Input: part model. Units: mm. Frame: model coordinates. Round coordinates to 2 decimals unless told otherwise and drop trailing zeros. Loops run counter-clockwise (first coordinate to the right, second up) from the corner with the lowest first, then second, coordinate; pieces in that order, holes last. Notation, with made-up numbers: (75, -16) -> (102, -16) arc R25 ccw to (102, 7) -> close; hole circle Ø6 at (86.25, 32). An arc over 180 degrees is marked (long way). Answer as a JSON object with one key per item and string values.
```python
from build123d import *

# Parameters (mm, degrees)
F0_W     = 15
F0_H     = 100
F2_R     = 3.9
F3_DEPTH = 10
F4_R     = 5


with BuildPart() as f1:
    # F0 (on Top) → F1 (revolve)
    with BuildSketch(Plane.XY):
        with Locations((-7.5, -50)):
            Rectangle(F0_W, F0_H)
    revolve(axis=Axis((0, -50, 0), (0, 1, 0)))

    # F2 (on face) → F3 (cut)
    with BuildSketch(Plane(origin=(0, 0, 0), x_dir=(-1, 0, 0), z_dir=(0, 1, 0))):
        Circle(F2_R)
    extrude(amount=-F3_DEPTH, mode=Mode.SUBTRACT)

    # F4
    f4_edges = [f1.edges().sort_by_distance(p)[0] for p in [
        (15, 0, 0),
        (15, -100, 0),
    ]]
    fillet(f4_edges, radius=F4_R)


solid = f1.part
```
1) Section A-A, the plane z = 0. Output: boundary loops of the cut face in (x, y), plus the area to 3 significant figures.
Output:
{"outline": "(-15, -95) arc R5 ccw to (-10, -100) -> (10, -100) arc R5 ccw to (15, -95) -> (15, -5) arc R5 ccw to (10, 0) -> (3.9, 0) -> (3.9, -10) -> (-3.9, -10) -> (-3.9, 0) -> (-10, 0) arc R5 ccw to (-15, -5) -> close", "area": "2,900 mm^2"}
2) Draft query along X for faces 1 (the face through (2.87, -4.93, 2.64)), 2 (the face through (0, -10, 0)), 3 (the face through (-4.3, 0, 0.1)), 4 (the face through (14.985, -49.37, 0.66)). Return one class per face: +X half, -X half, draft (parallel to the pull), parting line (faces both ways), or undercut.
Output:
{"face 1": "undercut", "face 2": "undercut", "face 3": "draft", "face 4": "parting line"}
3) Section C-C, the plane y = -60. Output: boundary loops of the cut face in (x, z).
Output:
{"outline": "circle Ø30 at (0, 0)"}
4) Section B-B, the plane x = 0. Output: boundary loops of the cut face in (y, z), plus the area to 3 significant figures.
Output:
{"outline": "(-100, -10) arc R5 ccw to (-95, -15) -> (-5, -15) arc R5 ccw to (0, -10) -> (0, -3.9) -> (-10, -3.9) -> (-10, 3.9) -> (0, 3.9) -> (0, 10) arc R5 ccw to (-5, 15) -> (-95, 15) arc R5 ccw to (-100, 10) -> close", "area": "2,900 mm^2"}
5) Ray query, probe 1 along Z at (x, y) = (0, -6.25); probe 2 along Z at (x, y) = (-0.5, -14.5); probe 3 along Z at (x, y) = (0, -3.75). Return the intervals inside material, ascending.
Output:
{"probe 1": "z = -15 to -3.9, 3.9 to 15", "probe 2": "z = -14.99 to 14.99", "probe 3": "z = -14.84 to -3.9, 3.9 to 14.84"}
6) Contact query for flat-ended pins moving along their axis: P1, Ø1, axis at x = 11.5, z = 5.5, coming from the -Y side; P2, Ø12, axis at x = 6.5, y = -69, coming from the -Z side; P3, Ø3, axis at x = -11, z = -10.5, coming from the -Y side. Output: stop coordinate, or through.
Output:
{"P1": "stops at y = -99.47", "P2": "stops at z = -14.99", "P3": "stops at y = -98.36"}
